```python
from build123d import *

# Parameters (mm, degrees)
BOSS_EXTRUDE1_DEPTH      = 152.4
BOSS_EXTRUDE1_DEPTH_BACK = 152.4
CUT_EXTRUDE1_DEPTH       = 157.875606199
LPATTERN1_COUNT          = 6
LPATTERN1_PITCH          = 50.8


with BuildPart() as part:
    # Sketch5 → Boss-Extrude1 (new, two sides: drawn at the far end of the back side and taken through both)
    with BuildSketch(Plane.XY.offset(-BOSS_EXTRUDE1_DEPTH_BACK)):
        with BuildLine():
            Line((-25.908, -20.6375), (27.4955, -20.6375))
            ThreePointArc((27.4955, -20.6375), (29.942619793, -19.623869793), (30.95625, -17.17675))
            Line((30.95625, -17.17675), (30.95625, 17.17675))
            ThreePointArc((30.95625, 17.17675), (29.942619793, 19.623869793), (27.4955, 20.6375))
            Line((27.4955, 20.6375), (-25.908, 20.6375))
            ThreePointArc((-25.908, 20.6375), (-29.477651808, 19.158901808), (-30.95625, 15.58925))
            Line((-30.95625, 15.58925), (-30.95625, 14.57325))
            ThreePointArc((-30.95625, 14.57325), (-29.942619793, 12.126130207), (-27.4955, 11.1125))
            Line((-27.4955, 11.1125), (-25.08885, 11.1125))
            ThreePointArc((-25.08885, 11.1125), (-23.81885, 12.3825), (-25.08885, 13.6525))
            Line((-25.08885, 13.6525), (-27.4955, 13.6525))
            ThreePointArc((-27.4955, 13.6525), (-28.146568569, 13.922181431), (-28.41625, 14.57325))
            Line((-28.41625, 14.57325), (-28.41625, 15.58925))
            ThreePointArc((-28.41625, 15.58925), (-27.681600584, 17.362850584), (-25.908, 18.0975))
            Line((-25.908, 18.0975), (27.4955, 18.0975))
            ThreePointArc((27.4955, 18.0975), (28.146568569, 17.827818569), (28.41625, 17.17675))
            Line((28.41625, 17.17675), (28.41625, -17.17675))
            ThreePointArc((28.41625, -17.17675), (28.146568569, -17.827818569), (27.4955, -18.0975))
            Line((27.4955, -18.0975), (-25.908, -18.0975))
            ThreePointArc((-25.908, -18.0975), (-27.681600584, -17.362850584), (-28.41625, -15.58925))
            Line((-28.41625, -15.58925), (-28.41625, -14.57325))
            ThreePointArc((-28.41625, -14.57325), (-28.146568569, -13.922181431), (-27.4955, -13.6525))
            Line((-27.4955, -13.6525), (-25.08885, -13.6525))
            ThreePointArc((-25.08885, -13.6525), (-23.81885, -12.3825), (-25.08885, -11.1125))
            Line((-25.08885, -11.1125), (-27.4955, -11.1125))
            ThreePointArc((-27.4955, -11.1125), (-29.942619793, -12.126130207), (-30.95625, -14.57325))
            Line((-30.95625, -14.57325), (-30.95625, -15.58925))
            ThreePointArc((-30.95625, -15.58925), (-29.477651808, -19.158901808), (-25.908, -20.6375))
        make_face()
    extrude(amount=BOSS_EXTRUDE1_DEPTH + BOSS_EXTRUDE1_DEPTH_BACK)

    # Sketch2 → Cut-Extrude1 (cut, through all)
    with BuildSketch(Plane(origin=(0, 0, 0), x_dir=(0, 0, -1), z_dir=(1, 0, 0))):
        with BuildLine():
            Line((-134.14375, 7.14375), (-119.85625, 7.14375))
            ThreePointArc((-119.85625, 7.14375), (-112.7125, 0), (-119.85625, -7.14375))
            Line((-119.85625, -7.14375), (-134.14375, -7.14375))
            ThreePointArc((-134.14375, -7.14375), (-141.2875, 0), (-134.14375, 7.14375))
        make_face()
    cut_extrude1 = extrude(amount=CUT_EXTRUDE1_DEPTH, mode=Mode.SUBTRACT)

    # LPattern1: Cut-Extrude1 ×6
    with Locations(*[(0, 0, -i * LPATTERN1_PITCH) for i in range(1, LPATTERN1_COUNT)]):
        add(cut_extrude1, mode=Mode.SUBTRACT)


solid = part.part
```
The model under review builds one solid part; all positions refer to its coordinate system, in mm. A direction names the side the tool comes from. Give positions to 0.01 mm unless a question says otherwise; leave off trailing zeros. Write each loop counter-clockwise with the first axis right and the second up, starting at its lowest first coordinate (ties: lowest second). Pieces come first, ordered by that corner, then holes. Notation, with made-up numbers: (-13.75, 64) - (23.25, 64) arc R12 cw to (23.25, 72) - close; hole circle Ø10 at (66.5, 83.25). An arc over 180 degrees is marked (long way). Answer in a Markdown table with one row per item. Add a question column.
1. Insertion check: P1, Ø1.3, axis at x = 30, z = -22.5, coming from the -Y side; P2, Ø3, axis at x = 30, z = -127, coming from the -Y side; P3, Ø2, axis at x = 30, z = 74, coming from the -Y side. Each pin has a flat end and moves straight along its axis. Give the tip position at first contact, or say it passes through.
2. We need section C-C on x = -12. Write out the cut boundary in (y, z).
3. Draft analysis for pull direction Z (two halves, no side actions). For faces 1 (the cylindrical face through (29.668, 0.157, -90.486)), 2 (the cylindrical face through (-29.517, -19.119, -2.134)), 3 (the flat face through (2.15, -18.25, 152.4)), 4 (the flat face through (2.15, -18.25, -152.4)), state which applies: +Z half, -Z half, draft (parallel to the pull), parting line (faces both ways), or undercut.
4. We need section A-A on y = 0. Write out the cut boundary in (x, z), then the cut area to 3 significant figures.
5. Tool access review of faces 5 (the flat face through (0, 18.098, -2)), 6 (the cylindrical face through (29.668, 0.157, 11.114)), 7 (the flat face through (1, 20.638, -2)): name each direction out of +Z, -Z, +X, -X, +Y, -Y from which nothing blocks a thin tool from reaching the whole face with its end or side.
6. Wall thickness on line 1 along Y through (x, z) = (-3, 105); line 2 along X through (y, z) = (-15, -83); line 3 along X through (y, z) = (-16, -107.5): over which ranges is each line inside the solid? List them lowest first. Write a range as [from, to].
Ans:
| question | item | result |
|---|---|---|
| 1 | P1 | stops at y = -20.1 |
| 1 | P2 | stops at y = -20.49 |
| 1 | P3 | stops at y = -20.29 |
| 2 | outline | (-20.64, -152.4) - (-18.1, -152.4) - (-18.1, 152.4) - (-20.64, 152.4) - close; (18.1, -152.4) - (20.64, -152.4) - (20.64, 152.4) - (18.1, 152.4) - close |
| 3 | face 1 | undercut |
| 3 | face 2 | draft |
| 3 | face 3 | +Z half |
| 3 | face 4 | -Z half |
| 4 | outline | (28.42, -152.4) - (30.96, -152.4) - (30.96, -141.29) - (28.42, -141.29) - close; (28.42, -112.71) - (30.96, -112.71) - (30.96, -90.49) - (28.42, -90.49) - close; (28.42, -61.91) - (30.96, -61.91) - (30.96, -39.69) - (28.42, -39.69) - close; (28.42, -11.11) - (30.96, -11.11) - (30.96, 11.11) - (28.42, 11.11) - close; (28.42, 39.69) - (30.96, 39.69) - (30.96, 61.91) - (28.42, 61.91) - close; (28.42, 90.49) - (30.96, 90.49) - (30.96, 112.71) - (28.42, 112.71) - close; (28.42, 141.29) - (30.96, 141.29) - (30.96, 152.4) - (28.42, 152.4) - close |
| 4 | area | 339 mm^2 |
| 5 | face 5 | +Z, -Z |
| 5 | face 6 | +X, -X |
| 5 | face 7 | +Z, -Z, +X, -X, +Y |
| 6 | line 1 | y = [-20.64, -18.1], [18.1, 20.64] |
| 6 | line 2 | x = [-30.96, -28.42], [28.42, 30.96] |
| 6 | line 3 | x = [-30.94, -28.38], [28.42, 30.96] |
